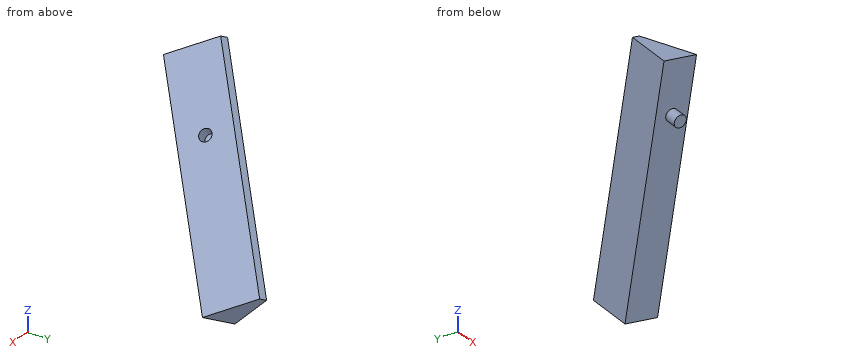
```python
from build123d import *

# Parameters (mm, degrees)
PAD001_DEPTH            = 150
SKETCH001_R             = 7.5
PAD_DEPTH               = 15
SKETCH003_R             = 7.5
POCKET003_DEPTH         = 15
BODY004_PLACEMENT_ANGLE = 180


with BuildPart() as part:
    # Sketch002 (on DatumPlane) → Pad001 (new body, symmetric)
    with BuildSketch(Plane(origin=(0, -50, 50), x_dir=(0.816497, -0.408248, -0.408248), z_dir=(-0.57735, -0.57735, -0.57735))):
        Polygon((0, 0), (0, 55.710678), (-8.660254, 55.710678), (-40.824829, 0), align=None)
    extrude(amount=PAD001_DEPTH, both=True)

    # Sketch001 (on Face7 of Binder001) → Pad (join)
    with BuildSketch(Plane(origin=(0, -50, 50), x_dir=(1, 0, 0), z_dir=(0, -0.707107, 0.707107))):
        with Locations((32.196959, 80.888716)):
            Circle(SKETCH001_R)
    extrude(amount=-PAD_DEPTH)

    # Sketch003 (on Face6 of Pad) → Pocket003 (cut)
    with BuildSketch(Plane(origin=(-25, -50, 75), x_dir=(-0.408248, 0.816497, -0.408248), z_dir=(-0.707107, 0, 0.707107))):
        with Locations((-11.75216, -47.456286)):
            Circle(SKETCH003_R)
    extrude(amount=-POCKET003_DEPTH, mode=Mode.SUBTRACT)


with BuildPart() as part_1:
    # Body004 placement: moved
    add(part.part.rotate(Axis((0, 0, 0), (0, 0, 1)), BODY004_PLACEMENT_ANGLE))


solid = part_1.part
```
Design review of the part built by this model. Coordinates are the model's own, in mm. Give positions to 0.01 mm unless a question says otherwise; leave off trailing zeros. Order: outer loops, then holes, each group sorted by start corner. A loop starts at its lowest first (then second) coordinate and runs counter-clockwise, first axis right, second up. Notation, with made-up numbers: (57.5, 54) - (63.5, 54) arc R21 ccw to (63.5, 63) - close; hole circle Ø11 at (48.25, 89.25). An arc over 180 degrees is marked (long way). Use a Markdown table: item, result. Add a question column.
(1) Clearance check with flat-ended pins moving along their axes: P1, Ø6, axis at y = 108.5, z = 54.5, coming from the -X side; P2, Ø2, axis at x = -11, y = 61.5, coming from the +Z side; P3, Ø6, axis at x = -36.5, z = 92, coming from the -Y side. State where each tip first meets the part, or that it passes through.
(2) Add section B-B on z = -8.5. Give the boundary of the cut face in (x, y).
(3) Add section C-C on y = 160. Give the boundary of the cut face in (x, z), then the cut area to 3 significant figures.
(4) Wall thickness on probe 1 along Z at (x, y) = (-55, -13.5); probe 2 along X at (y, z) = (22.5, 128); probe 3 along Z at (x, y) = (-8, 59.5): over which ranges is each line inside the solid? List them lowest first. Write a range as [from, to].
(5) Add section A-A on x = -59. Give the boundary of the cut face in (y, z), then the cut area to 3 significant figures.
Report:
| question | item | result |
|---|---|---|
| 1 | P1 | stops at x = 24.88 |
| 1 | P2 | stops at z = 112 |
| 1 | P3 | stops at y = -16.21 |
| 2 | outline | (58.5, 108.5) - (108.5, 108.5) - (108.5, 142.81) - (86.6, 164.71) - close |
| 3 | outline | (70.61, 18.79) - (86.6, -13.21) - (99.9, 0.1) - (81.21, 18.79) - close |
| 3 | area | 418 mm² |
| 4 | probe 1 | z = [113.5, 155] |
| 4 | probe 2 | x = [-52.75, -28] |
| 4 | probe 3 | z = [75.5, 108] |
| 5 | outline | (-50.4, 150.4) - (-9, 109) - (30.39, 148.39) - (19.79, 159) - (-41.81, 159) - close |
| 5 | area | 2,310 mm² |
